The listing builds one solid part. Answer for the finished solid, in the listing's coordinates (mm). Coordinates: 2 decimals unless noted, no trailing zeros. Write each loop counter-clockwise with the first axis right and the second up, starting at its lowest first coordinate (ties: lowest second). Pieces come first, ordered by that corner, then holes.
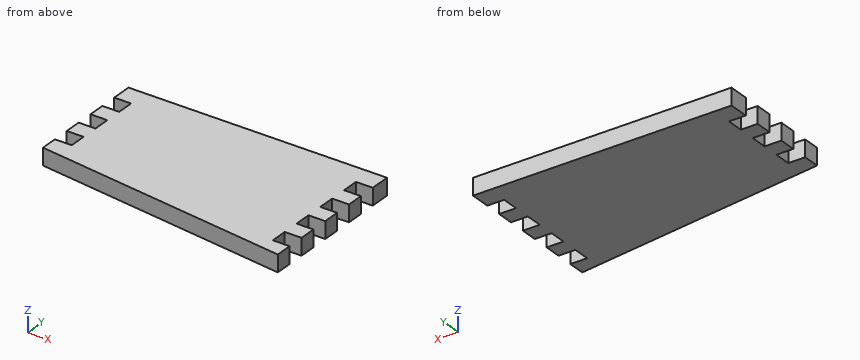
from build123d import *

# Parameters (mm, degrees)
F0_W     = 10
F0_H     = 10
F1_DEPTH = 10


# Not quite as in the source:
# - a feature names something its author has since deleted; it is built from what else it names


with BuildPart() as f1:
    # F0 (on Top) → F1 (new body)
    with BuildSketch(Plane.XY):
        Polygon((-2.2346749902, 36.9413525529), (-135.6346749902, 36.9413525529), (-135.6346749902, 26.9413525529), (-135.6346749902, 16.9413525529), (-135.6346749902, 6.9413525529), (-135.6346749902, -3.0586474471), (-135.6346749902, -13.0586474471), (-135.6346749902, -23.0586474471), (-135.6346749902, -33.0586474471), (-2.2346749902, -33.0586474471), (-2.2346749902, -23.0586474471), (-2.2346749902, -13.0586474471), (-2.2346749902, -3.0586474471), (-2.2346749902, 6.9413525529), (-2.2346749902, 16.9413525529), (-2.2346749902, 26.9413525529), align=None)
        with Locations((-140.6346749902, 31.9413525529)):
            Rectangle(F0_W, F0_H)
        with Locations((-140.6346749902, 11.9413525529)):
            Rectangle(F0_W, F0_H)
        with Locations((-140.6346749902, -8.0586474471)):
            Rectangle(F0_W, F0_H)
        with Locations((-140.6346749902, -28.0586474471)):
            Rectangle(F0_W, F0_H)
        with Locations((2.7653250098, 31.9413525529)):
            Rectangle(F0_W, F0_H)
        with Locations((2.7653250098, 11.9413525529)):
            Rectangle(F0_W, F0_H)
        with Locations((2.7653250098, -8.0586474471)):
            Rectangle(F0_W, F0_H)
        with Locations((2.7653250098, -28.0586474471)):
            Rectangle(F0_W, F0_H)
        Polygon((-135.6346749902, -33.0586474471), (-145.6346749902, -33.0586474471), (-2.2346749902, -51.7548664823), (-2.2346749902, -43.0586474471), (-2.2346749902, -33.0586474471), align=None)
        Polygon((-2.2346749902, -43.0586474471), (-2.2346749902, -51.7548664823), (7.7653250098, -53.0586474471), (7.7653250098, -43.0586474471), align=None)
        Polygon((-145.6346749902, 38.9413525529), (-145.6346749902, 36.9413525529), (-135.6346749902, 36.9413525529), (-2.2346749902, 36.9413525529), (7.7653250098, 36.9413525529), (7.7653250098, 38.9413525529), align=None)
    extrude(amount=F1_DEPTH)


solid = f1.part
1. Section B-B on y = 25 is taken. Give the vertices of the cut face in (x, z), then the cut area to 3 significant figures.
Results found:
outline: (-135.63, 0) - (-2.23, 0) - (-2.23, 10) - (-135.63, 10) - close
area: 1,330 mm2
2. Find the intervals of material crossed by L1, parallel to Y at x = 1, z = 5.25; L2, parallel to X at y = 5, z = 2.5; L3, parallel to Y at x = -0.5, z = 2.5, in increasing order.
Results found:
L1: y = -52.18 to -43.06, -33.06 to -23.06, -13.06 to -3.06, 6.94 to 16.94, 26.94 to 38.94
L2: x = -135.63 to -2.23
L3: y = -51.98 to -43.06, -33.06 to -23.06, -13.06 to -3.06, 6.94 to 16.94, 26.94 to 38.94
3. Flat-ended cylindrical pins translate along their axes: P1, Ø3, axis at y = 19.5, z = 3.5, coming from the -X side; P2, Ø3, axis at y = 20, z = 6, coming from the +X side; P3, Ø2, axis at x = -85.5, z = 3, coming from the -Y side. Find the tip coordinate at first contact, or state that the pin passes through.
Results found:
P1: stops at x = -135.63
P2: stops at x = -2.23
P3: stops at y = -41.03
4. Section C-C on x = -82.5 is taken. Give the vertices of the cut face in (y, z), then the cut area to 3 significant figures.
Results found:
outline: (-41.29, 0) - (38.94, 0) - (38.94, 10) - (-41.29, 10) - close
area: 802 mm2
